from build123d import *

# Parameters (mm, degrees)
F0_R     = 27
F0_R_2   = 25.5
F1_DEPTH = 15
F0_R_3   = 47
F2_DEPTH = 3
F3_W     = 16.0624054491
F3_H     = 1.5
F3_W_2   = 1.5
F3_H_2   = 16.0624054491
F4_DEPTH = 3
F5_DEPTH = 3


with BuildPart() as f1:
    # F0 (on Top) → F1 (new body)
    with BuildSketch(Plane.XY):
        Circle(F0_R)
        Circle(F0_R_2, mode=Mode.SUBTRACT)
    extrude(amount=F1_DEPTH)

    # F0 (on Top) → F2 (join)
    with BuildSketch(Plane.XY):
        Circle(F0_R_3)
        with BuildLine():
            ThreePointArc((-3, -42.8952211791), (-30.405591591, -30.405591591), (-42.8952211791, -3))
            Line((-42.8952211791, -3), (-32.8633534503, -3))
            ThreePointArc((-32.8633534503, -3), (-23.3345237792, -23.3345237792), (-3, -32.8633534503))
            Line((-3, -32.8633534503), (-3, -42.8952211791))
        make_face(mode=Mode.SUBTRACT)
        with BuildLine():
            ThreePointArc((3, -32.8633534503), (23.3345237792, -23.3345237792), (32.8633534503, -3))
            Line((32.8633534503, -3), (42.8952211791, -3))
            ThreePointArc((42.8952211791, -3), (30.405591591, -30.405591591), (3, -42.8952211791))
            Line((3, -42.8952211791), (3, -32.8633534503))
        make_face(mode=Mode.SUBTRACT)
        with BuildLine():
            ThreePointArc((-3, 32.8633534503), (-23.3345237792, 23.3345237792), (-32.8633534503, 3))
            Line((-32.8633534503, 3), (-42.8952211791, 3))
            ThreePointArc((-42.8952211791, 3), (-30.405591591, 30.405591591), (-3, 42.8952211791))
            Line((-3, 42.8952211791), (-3, 32.8633534503))
        make_face(mode=Mode.SUBTRACT)
        Circle(F0_R, mode=Mode.SUBTRACT)
        with BuildLine():
            Line((42.8952211791, 3), (32.8633534503, 3))
            ThreePointArc((32.8633534503, 3), (23.3345237792, 23.3345237792), (3, 32.8633534503))
            Line((3, 32.8633534503), (3, 42.8952211791))
            ThreePointArc((3, 42.8952211791), (30.405591591, 30.405591591), (42.8952211791, 3))
        make_face(mode=Mode.SUBTRACT)
    extrude(amount=F2_DEPTH)

    # F3 (on face) → F4 (join)
    with BuildSketch(Plane.XY.offset(3)):
        with Locations((-34.8640184545, 2.25)):
            Rectangle(F3_W, F3_H)
        with Locations((-34.8640184545, -2.25)):
            Rectangle(F3_W, F3_H)
        with Locations((34.8640184545, 2.25)):
            Rectangle(F3_W, F3_H)
        with Locations((34.8640184545, -2.25)):
            Rectangle(F3_W, F3_H)
        with Locations((-2.25, 34.8640184545)):
            Rectangle(F3_W_2, F3_H_2)
        with Locations((2.25, 34.8640184545)):
            Rectangle(F3_W_2, F3_H_2)
        with Locations((-2.25, -34.8640184545)):
            Rectangle(F3_W_2, F3_H_2)
        with Locations((2.25, -34.8640184545)):
            Rectangle(F3_W_2, F3_H_2)
    extrude(amount=F4_DEPTH)

    # F3 (on face) → F5 (join)
    with BuildSketch(Plane.XY.offset(3)):
        with Locations((-34.8640184545, 2.25)):
            Rectangle(F3_W, F3_H)
        with Locations((-34.8640184545, -2.25)):
            Rectangle(F3_W, F3_H)
        with Locations((34.8640184545, 2.25)):
            Rectangle(F3_W, F3_H)
        with Locations((34.8640184545, -2.25)):
            Rectangle(F3_W, F3_H)
        with Locations((-2.25, 34.8640184545)):
            Rectangle(F3_W_2, F3_H_2)
        with Locations((2.25, 34.8640184545)):
            Rectangle(F3_W_2, F3_H_2)
        with Locations((-2.25, -34.8640184545)):
            Rectangle(F3_W_2, F3_H_2)
        with Locations((2.25, -34.8640184545)):
            Rectangle(F3_W_2, F3_H_2)
    extrude(amount=-F5_DEPTH)


solid = f1.part
CAD build for the part. Positions are in the model's coordinates, mm. A direction names the side the tool comes from. Give positions to 0.01 mm unless a question says otherwise; leave off trailing zeros. Write each loop counter-clockwise with the first axis right and the second up, starting at its lowest first coordinate (ties: lowest second). Pieces come first, ordered by that corner, then holes. Notation, with made-up numbers: (-23.5, 61.5) - (18.5, 61.5) arc R22 cw to (18.5, 100.5) - close; hole circle Ø9 at (26.25, 21.5). An arc over 180 degrees is marked (long way). Put each result on its own line as item: value.
(1) Drop flat-ended pins along their axis: pin 1 Ø1.8 at (x, z) = (32.5, 3.5) entering from -Y; pin 2 Ø1 at (x, y) = (25.5, 37) entering from -Z; pin 3 Ø1.7 at (x, y) = (-33.5, 2) entering from +Z; pin 4 Ø5 at (y, z) = (-25.5, 7.5) entering from -X. Give the stop position or say it passes through.
Working result:
pin 1: y = -34.65
pin 2: z = 0
pin 3: z = 6
pin 4: x = -14.14
(2) Tool access for faces 1 (the flat face through (35, -1.5, 4)), 2 (the flat face through (3, 37, 3)), 3 (the cylindrical face through (30.71, -30.1, 1.48)), 4 (the flat face through (-1.5, -35, 4)): list every direction of +Z, -Z, +X, -X, +Y, -Y with a clear straight run to the whole face (end or side of a thin tool).
Working result:
face 1: +Z, +X
face 2: +Z
face 3: +Z, -Z
face 4: +Z, -Y
(3) Saw through at A-A (y = 0). List the corners of the cut face in (x, z).
Working result:
outline: (-47, 0) - (-25.5, 0) - (-25.5, 15) - (-27, 15) - (-27, 3) - (-47, 3) - close; (25.5, 0) - (47, 0) - (47, 3) - (27, 3) - (27, 15) - (25.5, 15) - close
(4) Saw through at D-D (x = 12). List the corners of the cut face in (y, z), then the cut area to 3 significant figures.
Working result:
outline: (-45.44, 0) - (-41.29, 0) - (-41.29, 3) - (-45.44, 3) - close; (-30.74, 0) - (-22.5, 0) - (-22.5, 15) - (-24.19, 15) - (-24.19, 3) - (-30.74, 3) - close; (22.5, 0) - (30.74, 0) - (30.74, 3) - (24.19, 3) - (24.19, 15) - (22.5, 15) - close; (41.29, 0) - (45.44, 0) - (45.44, 3) - (41.29, 3) - close
area: 115 mm^2
(5) Pull direction X, two halves, no side cores. Call faces 5 (the flat face through (-35, -1.5, 4)), 6 (the flat face through (37, -3, 3)): released by +X, released by -X, zero draft, split by the parting line, or undercut.
Working result:
face 5: zero draft
face 6: undercut
(6) Wall check: L1, parallel to X at y = 29.5, z = 5; L2, parallel to Y at x = 0, z = 8. Give the ranges that are in metal, low to high.
Working result:
L1: -3 to -1.5, 1.5 to 3
L2: -27 to -25.5, 25.5 to 27
